Check sheet for the modelled part. Datum: model origin and axes. Units: mm. Give positions to 0.01 mm unless a question says otherwise; leave off trailing zeros. Order: outer loops, then holes, each group sorted by start corner. A loop starts at its lowest first (then second) coordinate and runs counter-clockwise, first axis right, second up. Notation, with made-up numbers: (-22, -30) - (19, -30) arc R30 cw to (19, -2) - close; hole circle Ø7 at (12, 14). An arc over 180 degrees is marked (long way). Answer in a Markdown table with one row per item.
from build123d import *

# Parameters (mm, degrees)
F1_DEPTH = 61.171658
F2_T     = -2.54


with BuildPart() as f1:
    # F0 (on Top) → F1 (new body)
    with BuildSketch(Plane.XY):
        with BuildLine():
            ThreePointArc((-38.1, 0), (-26.940768, -26.940768), (0, -38.1))
            ThreePointArc((0, -38.1), (26.940768, -26.940768), (38.1, 0))
            ThreePointArc((38.1, 0), (26.940768, 26.940768), (0, 38.1))
            ThreePointArc((0, 38.1), (-26.940768, 26.940768), (-38.1, 0))
        make_face()
    extrude(amount=F1_DEPTH)

    # F2
    f2_openings = [f1.faces().sort_by_distance(p)[0] for p in [
        (0, 0, 61.171658),
    ]]
    offset(amount=F2_T, openings=f2_openings)


solid = f1.part
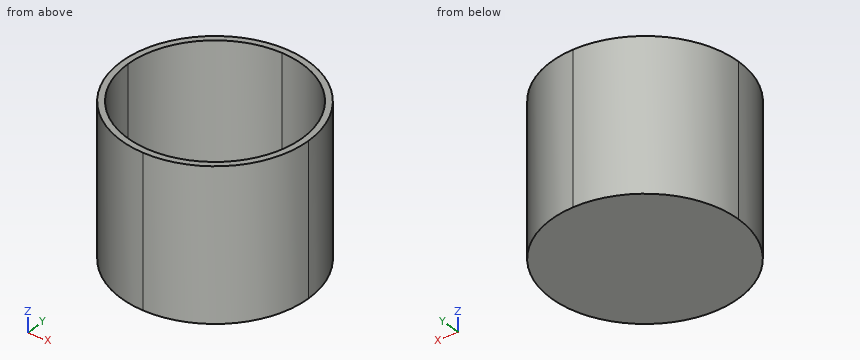
(1) Thickness scan on L1, parallel to Z at x = 1, y = 32.5; L2, parallel to X at y = 19, z = 52; L3, parallel to X at y = -4.5, z = 58. Record the ranges inside material, lowest first.
Geometry says:
| item | result |
|---|---|
| L1 | 0 to 2.54 |
| L2 | -33.02 to -30.06, 30.06 to 33.02 |
| L3 | -37.83 to -35.27, 35.27 to 37.83 |
(2) Cross-section at C-C, the plane x = 27.5. Record the cut outline in (y, z), then the cut area to 3 significant figures.
Geometry says:
| item | result |
|---|---|
| outline | (-26.37, 0) - (26.37, 0) - (26.37, 61.17) - (22.54, 61.17) - (22.54, 2.54) - (-22.54, 2.54) - (-22.54, 61.17) - (-26.37, 61.17) - close |
| area | 582 mm² |
(3) Cross-section at A-A, the plane z = 33.5. Record the cut outline in (x, y), then the cut area to 3 significant figures.
Geometry says:
| item | result |
|---|---|
| outline | (-38.1, 0) arc R38.1 ccw to (0, -38.1) arc R38.1 ccw to (38.1, 0) arc R38.1 ccw to (0, 38.1) arc R38.1 ccw to start; hole (-35.56, 0) arc R35.56 ccw to (0, -35.56) arc R35.56 ccw to (35.56, 0) arc R35.56 ccw to (0, 35.56) arc R35.56 ccw to start |
| area | 588 mm² |
(4) Cross-section at B-B, the plane y = 11. Record the cut outline in (x, z).
Geometry says:
| item | result |
|---|---|
| outline | (-36.48, 0) - (36.48, 0) - (36.48, 61.17) - (33.82, 61.17) - (33.82, 2.54) - (-33.82, 2.54) - (-33.82, 61.17) - (-36.48, 61.17) - close |
(5) Gauge pin test, flat ends, axial feed: P1, Ø3, axis at x = -6, z = 32.5, coming from the +Y side; P2, Ø1.5, axis at x = 7.5, y = 22, coming from the +Z side; P3, Ø6, axis at y = -5.5, z = 54.5, coming from the +X side. Record the tip position at first contact, or that the pin passes through.
Geometry says:
| item | result |
|---|---|
| P1 | y = 37.83 |
| P2 | z = 2.54 |
| P3 | x = 38.02 |
